```python
from build123d import *

# Parameters (mm, degrees)
BOX_W           = 833
BOX_H           = 61
BOX_DEPTH       = 19
FILLET_R        = 1
FILLET001_R     = 1
SKETCH_W        = 20
SKETCH_H        = 63
POCKET_DEPTH    = 5
SKETCH001_W     = 20
SKETCH001_H     = 63
POCKET001_DEPTH = 5
FILLET002_R     = 1


with BuildPart() as part:
    # Box → Box (new body)
    with BuildSketch(Plane.XY):
        with Locations((416.5, 30.5)):
            Rectangle(BOX_W, BOX_H)
    extrude(amount=BOX_DEPTH)

    # Fillet
    fillet_edges = [part.edges().sort_by_distance(p)[0] for p in [
        (416.5, 0, 19),
    ]]
    fillet(fillet_edges, radius=FILLET_R)

    # Fillet001
    fillet001_edges = [part.edges().sort_by_distance(p)[0] for p in [
        (833, 31, 19),
    ]]
    fillet(fillet001_edges, radius=FILLET001_R)

    # Sketch (on Face5 of Fillet001) → Pocket (cut)
    with BuildSketch(Plane(origin=(0, 0, 0), x_dir=(1, 0, 0), z_dir=(0, 0, -1))):
        with Locations((10, -31.5)):
            Rectangle(SKETCH_W, SKETCH_H)
    extrude(amount=-POCKET_DEPTH, mode=Mode.SUBTRACT)

    # Sketch001 (on Face6 of Pocket) → Pocket001 (cut)
    with BuildSketch(Plane(origin=(0, 0, 0), x_dir=(1, 0, 0), z_dir=(0, 0, -1))):
        with Locations((823, -31.5)):
            Rectangle(SKETCH001_W, SKETCH001_H)
    extrude(amount=-POCKET001_DEPTH, mode=Mode.SUBTRACT)

    # Fillet002
    fillet002_edges = [part.edges().sort_by_distance(p)[0] for p in [
        (0, 0, 11.5),
    ]]
    fillet(fillet002_edges, radius=FILLET002_R)


solid = part.part
```
Work out the finished part from the listing and answer in its coordinate system (mm). A direction names the side the tool comes from. Round coordinates to 2 decimals unless told otherwise and drop trailing zeros.
(1) For faces 1 (the flat face through (10, 30, 5)), 2 (the flat face through (411, 31, 0)), 3 (the flat face through (823, 30, 5)), determine the directions among +Z, -Z, +X, -X, +Y, -Y from which every point of the face is accessible in a straight line to the end or side of a thin tool.
Computed values:
face 1: -Z, -X, +Y, -Y
face 2: -Z, +X, -X, +Y, -Y
face 3: -Z, +X, +Y, -Y
(2) Each of these flat-tipped pins is pushed along its axis until it touches: P1, Ø16, axis at x = 6.5, y = 17, coming from the -Z side; P2, Ø5, axis at x = 667.5, y = 34, coming from the -Z side; P3, Ø2.5, axis at y = 25, z = 1.5, coming from the -X side. Where does it stop, or does it pass through?
Computed values:
P1: stops at z = 5
P2: stops at z = 0
P3: stops at x = 20
(3) Find the intervals of material crossed by L1, parallel to X at y = 34, z = 2, in increasing order.
Computed values:
L1: x = 20 to 813
